Build history of the part. All positions in model axes, mm. Face numbers are marked on the shaded views. A direction names the side the tool comes from. Round coordinates to 2 decimals unless told otherwise and drop trailing zeros. Write each loop counter-clockwise with the first axis right and the second up, starting at its lowest first coordinate (ties: lowest second). Pieces come first, ordered by that corner, then holes. Notation, with made-up numbers: (-1.5, -2.5) - (51.5, -2.5) arc R20 ccw to (51.5, 17.5) - close; hole circle Ø3 at (-28.5, -20). An arc over 180 degrees is marked (long way). Answer as a JSON object with one key per item and string values. Group by question number.
Item 1: Slice it at C-C, the plane x = 57. List the corners of the cut face in (y, z).
Item 2: Slice it at B-B, the plane z = 36.5. List the corners of the cut face in (x, y), then the cut area to 4 significant figures.
Item 3: Which spindle directions (+Z, -Z, +X, -X, +Y, -Y) get a long thin tool onto all of the face, cutting with end or side? Do the marked faces 1, 2, 3, 4 and 5. Say none if no direction does.
Item 4: Slice it at A-A, the plane x = 25. Give the number of separate pieces and of enclosed holes in the cut face, then the cut area to 3 significant figures.
Item 5: Flat gauge pins, fed straight in: pin 1 (3 mm diameter, centred on x = 75, y = 35, fed in from -Z); pin 2 (3.5 mm diameter, centred on x = 97, y = 39, fed in from +Z); pin 3 (2 mm diameter, centred on y = 51, z = 29, fed in from -X); pin 4 (8 mm diameter, centred on y = 51.5, z = 12.5, fed in from -X). Where does each tip first touch, or does it go through?
Item 6: Probe line 1 (Y direction, x = 25, z = 0.75); line 2 (X direction, y = 35, z = 0.7); line 3 (Z direction, x = 28.5, y = 69.5). List the from-to ranges inside material, lowest first. Write a range as from..to.
Item 7: Two-plate mould, pull along X, no slides. Class the marked faces 6, 7 and 8: +X half, -X half, draft (parallel to the pull), parting line (faces both ways), or undercut.
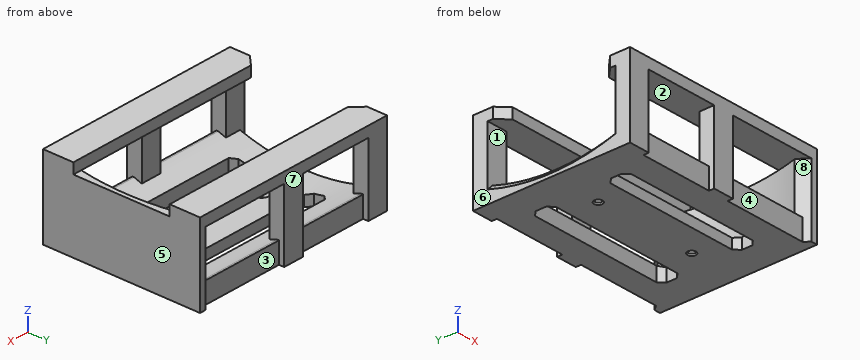
from build123d import *

# Parameters (mm, degrees)
CYLINDER001_R     = 120
CYLINDER001_DEPTH = 40
BOX001_W          = 10
BOX001_H          = 75
BOX001_DEPTH      = 34
CHAMFER004_SIZE   = 5
BOX008_W          = 70
BOX008_H          = 10
BOX008_DEPTH      = 10
CHAMFER_SIZE      = 2.5
BOX009_W          = 70
BOX009_H          = 10
BOX009_DEPTH      = 10
CHAMFER001_SIZE   = 2.5
CYLINDER005_R     = 2
CYLINDER005_DEPTH = 10
CYLINDER004_R     = 4
CYLINDER004_DEPTH = 10
CYLINDER003_R     = 2
CYLINDER003_DEPTH = 10
CYLINDER002_R     = 4
CYLINDER002_DEPTH = 10
CYLINDER_R        = 100
CYLINDER_DEPTH    = 100
BOX_W             = 100
BOX_H             = 70
BOX_DEPTH         = 10
CHAMFER012_SIZE   = 2.5
BOX002_W          = 10
BOX002_H          = 7
BOX002_DEPTH      = 34
BOX003_W          = 100
BOX003_H          = 14.5
BOX003_DEPTH      = 5
BOX004_W          = 10
BOX004_H          = 7
BOX004_DEPTH      = 34
BOX005_W          = 10
BOX005_H          = 7
BOX005_DEPTH      = 34
BOX006_W          = 10
BOX006_H          = 7
BOX006_DEPTH      = 34
BOX007_W          = 100
BOX007_H          = 14.5
BOX007_DEPTH      = 5
CHAMFER013_SIZE   = 5


with BuildPart() as cylinder001:
    # Cylinder001 → Cylinder001 (new body)
    with BuildSketch(Plane(origin=(-22, 35, 0), x_dir=(1, 0, 0), z_dir=(0, 0, 1))):
        Circle(CYLINDER001_R)
    extrude(amount=CYLINDER001_DEPTH)


with BuildPart() as chamfer004:
    # Box001 → Box001 (new body)
    with BuildSketch(Plane(origin=(90, -2.5, 0), x_dir=(1, 0, 0), z_dir=(0, 0, 1))):
        with Locations((5, 37.5)):
            Rectangle(BOX001_W, BOX001_H)
    extrude(amount=BOX001_DEPTH)

    # Cut001: cut Cylinder001
    add(cylinder001.part, mode=Mode.SUBTRACT)

    # Chamfer004
    chamfer004_edges = [chamfer004.edges().sort_by_distance(p)[0] for p in [
        (91.990131, -2.5, 17),
        (91.990131, 72.5, 17),
    ]]
    chamfer(chamfer004_edges, length=CHAMFER004_SIZE)


with BuildPart() as chamfer_body:
    # Box008 → Box008 (new body)
    with BuildSketch(Plane.XY):
        with Locations((35, 5)):
            Rectangle(BOX008_W, BOX008_H)
    extrude(amount=BOX008_DEPTH)

    # Chamfer
    chamfer_edges = [chamfer_body.edges().sort_by_distance(p)[0] for p in [
        (0, 0, 5),
        (0, 10, 5),
        (70, 0, 5),
        (70, 10, 5),
    ]]
    chamfer(chamfer_edges, length=CHAMFER_SIZE)


with BuildPart() as chamfer_body_1:
    # Chamfer placement: moved
    add(chamfer_body.part.moved(Location((15, 12.5, 0))))


with BuildPart() as fusion004:
    # Box009 → Box009 (new body)
    with BuildSketch(Plane.XY):
        with Locations((35, 5)):
            Rectangle(BOX009_W, BOX009_H)
    extrude(amount=BOX009_DEPTH)

    # Chamfer001
    chamfer001_edges = [fusion004.edges().sort_by_distance(p)[0] for p in [
        (0, 0, 5),
        (0, 10, 5),
        (70, 0, 5),
        (70, 10, 5),
    ]]
    chamfer(chamfer001_edges, length=CHAMFER001_SIZE)


with BuildPart() as fusion004_1:
    # Chamfer001 placement: moved
    add(fusion004.part.moved(Location((15, 48.5, 0))))

    # Fusion004: union Chamfer body
    add(chamfer_body_1.part)


with BuildPart() as cone001:
    # Cone001 → Cone001 (revolve)
    with BuildSketch(Plane(origin=(0, 35, 10), x_dir=(1, 0, 0), z_dir=(0, -1, 0))):
        Polygon((0, 0), (2, 0), (4, 3), (0, 3), align=None)
    revolve(axis=Axis((0, 35, 10), (0, 0, 1)))


with BuildPart() as cylinder005:
    # Cylinder005 → Cylinder005 (new body)
    with BuildSketch(Plane(origin=(0, 35, 0), x_dir=(1, 0, 0), z_dir=(0, 0, 1))):
        Circle(CYLINDER005_R)
    extrude(amount=CYLINDER005_DEPTH)


with BuildPart() as countersink_mount001:
    # Cylinder004 → Cylinder004 (new body)
    with BuildSketch(Plane(origin=(0, 35, 13), x_dir=(1, 0, 0), z_dir=(0, 0, 1))):
        Circle(CYLINDER004_R)
    extrude(amount=CYLINDER004_DEPTH)

    # Fusion001: union Cone001, Cylinder005
    add(cone001.part)
    add(cylinder005.part)


with BuildPart() as countersink_mount001_1:
    # Fusion001 placement: moved
    add(countersink_mount001.part.moved(Location((75, 0, -9))))


with BuildPart() as cone:
    # Cone → Cone (revolve)
    with BuildSketch(Plane(origin=(0, 35, 10), x_dir=(1, 0, 0), z_dir=(0, -1, 0))):
        Polygon((0, 0), (2, 0), (4, 3), (0, 3), align=None)
    revolve(axis=Axis((0, 35, 10), (0, 0, 1)))


with BuildPart() as cylinder003:
    # Cylinder003 → Cylinder003 (new body)
    with BuildSketch(Plane(origin=(0, 35, 0), x_dir=(1, 0, 0), z_dir=(0, 0, 1))):
        Circle(CYLINDER003_R)
    extrude(amount=CYLINDER003_DEPTH)


with BuildPart() as fusion002:
    # Cylinder002 → Cylinder002 (new body)
    with BuildSketch(Plane(origin=(0, 35, 13), x_dir=(1, 0, 0), z_dir=(0, 0, 1))):
        Circle(CYLINDER002_R)
    extrude(amount=CYLINDER002_DEPTH)

    # Fusion: union Cone, Cylinder003
    add(cone.part)
    add(cylinder003.part)


with BuildPart() as fusion002_1:
    # Fusion placement: moved
    add(fusion002.part.moved(Location((25, 0, -9))))

    # Fusion002: union countersink mount001
    add(countersink_mount001_1.part)


with BuildPart() as cylinder:
    # Cylinder → Cylinder (new body)
    with BuildSketch(Plane(origin=(0, 35, 104), x_dir=(0, 0, -1), z_dir=(1, 0, 0))):
        Circle(CYLINDER_R)
    extrude(amount=CYLINDER_DEPTH)


with BuildPart() as chamfer012:
    # Box → Box (new body)
    with BuildSketch(Plane.XY):
        with Locations((50, 35)):
            Rectangle(BOX_W, BOX_H)
    extrude(amount=BOX_DEPTH)

    # Cut: cut Cylinder
    add(cylinder.part, mode=Mode.SUBTRACT)

    # Cut002: cut Fusion002
    add(fusion002_1.part, mode=Mode.SUBTRACT)

    # Cut003: cut Fusion004
    add(fusion004_1.part, mode=Mode.SUBTRACT)

    # Chamfer012
    chamfer012_edges = [chamfer012.edges().sort_by_distance(p)[0] for p in [
        (0, 17.679492, 5.511422),
        (0, 52.320508, 5.511422),
    ]]
    chamfer(chamfer012_edges, length=CHAMFER012_SIZE)


with BuildPart() as cube002:
    # Box002 → Box002 (new body)
    with BuildSketch(Plane(origin=(0, 65.5, 0), x_dir=(1, 0, 0), z_dir=(0, 0, 1))):
        with Locations((5, 3.5)):
            Rectangle(BOX002_W, BOX002_H)
    extrude(amount=BOX002_DEPTH)


with BuildPart() as cube003:
    # Box003 → Box003 (new body)
    with BuildSketch(Plane(origin=(0, 58, 34), x_dir=(1, 0, 0), z_dir=(0, 0, 1))):
        with Locations((50, 7.25)):
            Rectangle(BOX003_W, BOX003_H)
    extrude(amount=BOX003_DEPTH)


with BuildPart() as cube004:
    # Box004 → Box004 (new body)
    with BuildSketch(Plane(origin=(45, 65.5, 0), x_dir=(1, 0, 0), z_dir=(0, 0, 1))):
        with Locations((5, 3.5)):
            Rectangle(BOX004_W, BOX004_H)
    extrude(amount=BOX004_DEPTH)


with BuildPart() as cube005:
    # Box005 → Box005 (new body)
    with BuildSketch(Plane(origin=(0, -2.5, 0), x_dir=(1, 0, 0), z_dir=(0, 0, 1))):
        with Locations((5, 3.5)):
            Rectangle(BOX005_W, BOX005_H)
    extrude(amount=BOX005_DEPTH)


with BuildPart() as cube006:
    # Box006 → Box006 (new body)
    with BuildSketch(Plane(origin=(45, -2.5, 0), x_dir=(1, 0, 0), z_dir=(0, 0, 1))):
        with Locations((5, 3.5)):
            Rectangle(BOX006_W, BOX006_H)
    extrude(amount=BOX006_DEPTH)


with BuildPart() as chamfer013:
    # Box007 → Box007 (new body)
    with BuildSketch(Plane(origin=(0, -2.5, 34), x_dir=(1, 0, 0), z_dir=(0, 0, 1))):
        with Locations((50, 7.25)):
            Rectangle(BOX007_W, BOX007_H)
    extrude(amount=BOX007_DEPTH)

    # Fusion003: union Cube002, Cube003, Cube004, Cube005, Cube006
    add(cube002.part)
    add(cube003.part)
    add(cube004.part)
    add(cube005.part)
    add(cube006.part)

    # Fusion005: union Chamfer004, Chamfer012
    add(chamfer004.part)
    add(chamfer012.part)

    # Chamfer013
    chamfer013_edges = [chamfer013.edges().sort_by_distance(p)[0] for p in [
        (0, 12, 36.5),
        (0, 58, 36.5),
    ]]
    chamfer(chamfer013_edges, length=CHAMFER013_SIZE)


solid = chamfer013.part
Geometry says:
{
 "1": {"outline": "(-2.5, 34) - (12, 34) - (12, 39) - (-2.5, 39) - close; (0, 0) - (12.5, 0) - (12.5, 6.56) arc R100 cw to (0.88, 10) - (0, 10) - close; (22.5, 0) - (48.5, 0) - (48.5, 4.92) arc R100 cw to (22.5, 4.78) - close; (58, 34) - (72.5, 34) - (72.5, 39) - (58, 39) - close; (58.5, 0) - (70, 0) - (70, 10) - (69.12, 10) arc R100 cw to (58.5, 6.8) - close"},
 "2": {"outline": "(0, -2.5) - (100, -2.5) - (100, 12) - (5, 12) - (0, 7) - close; (0, 63) - (5, 58) - (100, 58) - (100, 72.5) - (0, 72.5) - close", "area": "2,875 mm^2"},
 "3": {"face 1": "-X", "face 2": "none", "face 3": "-Z, +Y", "face 4": "-Z, -Y", "face 5": "+Z, -Z, +X, +Y, -Y"},
 "4": {"separate pieces": "6", "enclosed holes": "0", "area": "435 mm^2"},
 "5": {"pin 1": "passes through", "pin 2": "stops at z = 34", "pin 3": "stops at x = 96.79", "pin 4": "stops at x = 96.24"},
 "6": {"line 1": "y = 0..12.5, 22.5..33, 37..48.5, 58.5..70", "line 2": "x = 0..23, 27..73, 77..100", "line 3": "z = 0..10, 34..39"},
 "7": {"face 6": "-X half", "face 7": "draft", "face 8": "undercut"}
}
